Here's how the part is built. I have some questions about the finished solid (model axes, mm). Face numbers are marked on the shaded views. Give positions to 0.01 mm unless a question says otherwise; leave off trailing zeros. Order: outer loops, then holes, each group sorted by start corner. A loop starts at its lowest first (then second) coordinate and runs counter-clockwise, first axis right, second up.
Autodesk Inventor part; units mm, degrees
ref_plane "YZ Plane" through (0, 0, 0) normal (1, 0, 0) x (0, 1, 0)
ref_plane "XZ Plane" through (0, 0, 0) normal (0, 1, 0) x (-1, 0, 0)
ref_plane "XY Plane" through (0, 0, 0) normal (0, 0, 1) x (1, 0, 0)
sketch "Sketch1" plane through (0, 0, 0) normal (1, 0, 0) x (0, 1, 0)
  line L0 (12.7, 12.2788) -> (-12.7, 12.2788)
  line L1 (-12.7, 12.2788) -> (-12.7, -13.1212)
  line L2 (-12.7, -13.1212) -> (12.7, -13.1212)
  line L3 (12.7, -13.1212) -> (12.7, 12.2788)
  line L4 (0, 32.4321) -> (0, -31.5519)
  line L5 (24.3369, 0) -> (-19.9975, 0)
  point P0 (0, 0)
  dimension "d0" = 25.4
extrude "Extrusion1" add sketch "Sketch1" along normal blind 355.6
sketch "Sketch3" plane through (355.6, 0, 0) normal (1, 0, 0) x (0, 0, -1)
  line L0 (-10.6786, 11.1125) -> (11.521, 11.1125)
  line L1 (11.521, 11.1125) -> (11.521, -11.0998)
  line L2 (11.521, -11.0998) -> (-10.6786, -11.0998)
  line L3 (-10.6786, -11.0998) -> (-10.6786, 11.1125)
  line L4 (13.1212, 12.7) -> (-12.2788, 12.7)
  line L5 (-12.2788, 12.7) -> (-12.2788, -12.7)
  line L6 (13.1212, -12.7) -> (13.1212, 12.7)
  line L7 (-12.2788, -12.7) -> (13.1212, -12.7)
  point P0 (0, 0)
  dimension "d5" = 1.5875
  dimension "d6" = 1.6002
  dimension "d7" = 1.6002
  dimension "d8" = 1.6002
extrude "Extrusion2" cut sketch "Sketch3" against normal blind 279.4 contours L0 L1 L2 L3
sketch "Sketch4" plane through (0, -12.7, 12.2788) normal (0, 0, 1) x (1, 0, 0)
  circle A0 centre (342.9, 12.7) radius 3.175
  line L0 (355.6, 25.4) -> (355.6, 0)
  circle A1 centre (12.7, 12.7) radius 2.5781
  circle A2 centre (38.1, 12.7) radius 2.5781
  line L1 (0, 25.4) -> (355.6, 25.4)
  line L2 (0, 25.4) -> (0, 0)
  point P0 (0, 12.7)
  dimension "d11" = 6.35
  dimension "d12" = 12.7
  dimension "d15" = 5.1562
  dimension "d16" = 5.1562
  dimension "d17" = 25.4
  dimension "d18" = 12.7
  dimension "d19" = 12.7
  dimension "d20" = 12.7
extrude "Extrusion3" cut sketch "Sketch4" against normal blind 25.4
sketch "Sketch5" plane through (0, -12.7, 12.2788) normal (0, 0, 1) x (1, 0, 0)
  point P0 (0, 12.7)
equation "\"d19\" = d18"
properties part number "Part1-17-13.31255in" material "Aluminum 6061"
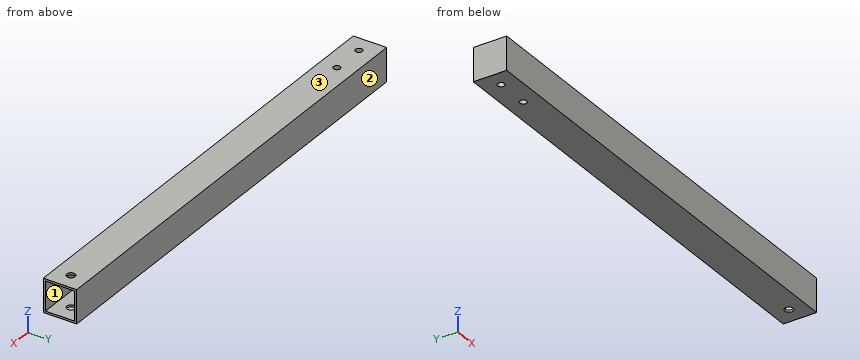
Q1. If we section it at A-A on z = -3: List the corners of the cut face in (x, y) for me.
Filled sheet:
outline: (0, -12.7) - (355.6, -12.7) - (355.6, -11.1) - (76.2, -11.1) - (76.2, 11.11) - (355.6, 11.11) - (355.6, 12.7) - (0, 12.7) - close; hole circle Ø5.16 at (12.7, 0); hole circle Ø5.16 at (38.1, 0)
Q2. If we section it at B-B on x = 342.9: List the corners of the cut face in (y, z) for me (1 decimal), plus the area to 3 significant figures.
Filled sheet:
outline: (-12.7, -13.1) - (-3.2, -13.1) - (-3.2, -11.5) - (-11.1, -11.5) - (-11.1, 10.7) - (-3.2, 10.7) - (-3.2, 12.3) - (-12.7, 12.3) - close; (3.2, -13.1) - (12.7, -13.1) - (12.7, 12.3) - (3.2, 12.3) - (3.2, 10.7) - (11.1, 10.7) - (11.1, -11.5) - (3.2, -11.5) - close
area: 132 mm2
Q3. Thinking about a two-plate mould opening in Y: for the marked faces 1, 2 and 3, which applies, released by +Y, released by -Y, zero draft, split by the parting line, or undercut?
Filled sheet:
face 1: undercut
face 2: released by +Y
face 3: zero draft
Q4. I need wall thicknesses on L1, parallel to X at y = -0.25, z = 10.75; L2, parallel to Z at x = 139, y = -0.75; L3, parallel to Y at x = 204.5, z = 10.25. Which ranges of each line are inside material? Lowest first, please.
Filled sheet:
L1: x = 0 to 10.13, 15.27 to 35.53, 40.67 to 339.73, 346.07 to 355.6
L2: z = -13.12 to -11.52, 10.68 to 12.28
L3: y = -12.7 to -11.1, 11.11 to 12.7
Q5. If we section it at C-C on x = 189.5: List the corners of the cut face in (y, z) for me, plus the area to 3 significant figures.
Filled sheet:
outline: (-12.7, -13.12) - (12.7, -13.12) - (12.7, 12.28) - (-12.7, 12.28) - close; hole (-11.1, -11.52) - (11.11, -11.52) - (11.11, 10.68) - (-11.1, 10.68) - close
area: 152 mm2
Q6. I'm going to push a flat-ended pin straight in: P1, Ø6, axis at y = 7, z = -5.5, coming from the +X side. Where does the tip first touch, or does it pass through?
Filled sheet:
P1: stops at x = 76.2
